Geometry check sheet. Reference: the model listing, model coordinates, mm. Coordinates: 2 decimals unless noted, no trailing zeros. Put each result on its own line as item: value. Start each with the question number.
1) Gauge pin test, flat ends, axial feed: pin 1 (1.5 mm diameter, centred on y = -1.5, z = 16.5, fed in from -X); pin 2 (3 mm diameter, centred on x = 17.8, z = 0, fed in from +Y); pin 3 (3 mm diameter, centred on x = 6.81, z = -16.45, fed in from -Y). Record the tip position at first contact, or that the pin passes through.
2) Cross-section at A-A on z = 0. Count the separate pieces of the cut face and the enclosed holes in it, plus the area to 3 significant figures.
3) Scan lines: line 1 along Z through (x, y) = (15, -0.85); line 2 along X through (y, z) = (-1.15, 17.5); line 3 along Z through (x, y) = (17.8, -1.45). Record each from-to range of solid material in increasing order.
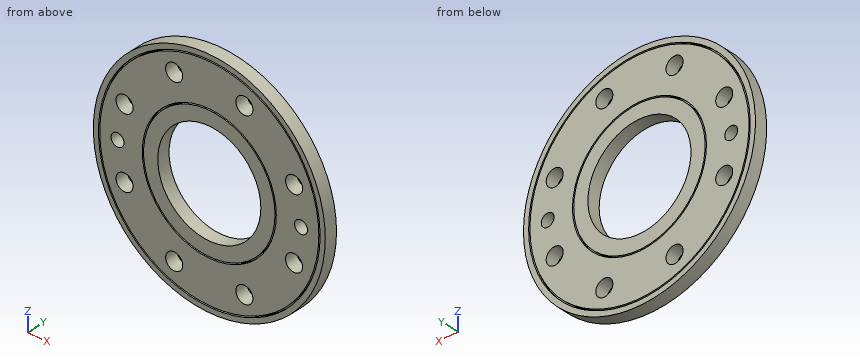
from build123d import *

# Parameters (mm, degrees)
F0_R     = 22.5
F0_R_2   = 10
F1_DEPTH = 2.5
F2_D     = 3.3
F3_D     = 2.5
F4_R     = 21.5
F4_R_2   = 21.25
F4_R_3   = 13
F4_R_4   = 12.75
F5_DEPTH = 0.5
F6_R     = 21.5
F6_R_2   = 21.25
F6_R_3   = 13
F6_R_4   = 12.75
F7_DEPTH = 0.5


with BuildPart() as f1:
    # F0 (on Front) → F1 (new body)
    with BuildSketch(Plane.XZ):
        Circle(F0_R)
        Circle(F0_R_2, mode=Mode.SUBTRACT)
    extrude(amount=F1_DEPTH)

    # F2 (through all)
    with Locations(Plane(origin=(0, 0, 0), x_dir=(1, 0, 0), z_dir=(0, 1, 0))):
        with Locations((-16.4450556787, -6.8117650961), (-6.8117650961, -16.4450556787), (6.8117650961, -16.4450556787), (16.4450556787, -6.8117650961), (16.4450556787, 6.8117650961), (6.8117650961, 16.4450556787), (-6.8117650961, 16.4450556787), (-16.4450556787, 6.8117650961)):
            Hole(F2_D / 2)

    # F3 (through all)
    with Locations(Plane(origin=(0, 0, 0), x_dir=(1, 0, 0), z_dir=(0, 1, 0))):
        with Locations((-17.8, 0), (17.8, 0)):
            Hole(F3_D / 2)

    # F4 (on face) → F5 (cut)
    with BuildSketch(Plane.XZ.offset(2.5)):
        Circle(F4_R)
        Circle(F4_R_2, mode=Mode.SUBTRACT)
        Circle(F4_R_3)
        Circle(F4_R_4, mode=Mode.SUBTRACT)
    extrude(amount=-F5_DEPTH, mode=Mode.SUBTRACT)

    # F6 (on face) → F7 (cut)
    with BuildSketch(Plane.XZ):
        Circle(F6_R)
        Circle(F6_R_2, mode=Mode.SUBTRACT)
        Circle(F6_R_3)
        Circle(F6_R_4, mode=Mode.SUBTRACT)
    extrude(amount=F7_DEPTH, mode=Mode.SUBTRACT)


solid = f1.part
Answer key:
1. pin 1: stops at x = -16.07
1. pin 2: stops at y = 0
1. pin 3: passes through
2. separate pieces: 4
2. enclosed holes: 0
2. area: 49.0 mm²
3. line 1: z = -16.77 to -7.61, -6.02 to 6.02, 7.61 to 16.77
3. line 2: x = -14.14 to -8.08, -5.54 to 5.54, 8.08 to 14.14
3. line 3: z = -13.76 to -7.75, -5.87 to -1.25, 1.25 to 5.87, 7.75 to 13.76
